Solid Edge part; units mm, degrees
sketch "Sketch1" plane through (0, 0, 0) normal (0, 0, 1) x (1, 0, 0)
  line L0 (0, 0) -> (-71.445, 0)
  line L1 (-40, -28.2156) -> (-71.445, 0)
  line L2 (-40, -52.2156) -> (-40, -28.2156)
  line L3 (-40, -52.2156) -> (-25, -52.2156)
  line L4 (-25, -52.2156) -> (-25, -165)
  line L5 (-25, -165) -> (0, -165)
  line L6 (0, -165) -> (0, 0)
  dimension "D1" = 40
  dimension "D2" = 25
  dimension "D3" = 40
extrude "Protrusion1" add sketch "Sketch1" along normal blind 12
sketch "Sketch2" plane through (0, -70, 6) normal (1, 0, 0) x (0, 1, 0)
  line L0 (70, 2) -> (-55, -6)
  line L1 (-55, -6) -> (-95, 2)
  dimension "D1" = 70
extrude "Extrusionsausschnitt_1" cut sketch "Sketch2" against normal blind 220 material side at (0, -62.4968, 3.9501)
mirror "Mirror1" about plane through (0, 0, 0) normal (-1, 0, 0) of "Protrusion1", "Extrusionsausschnitt_1"
chamfer "Fase_2" distance 2.5 angle 45 12 edges at (25, -88.6078, 2.3291) (25, -145, 4) (0, -165, 8) (-25, -145, 4) (-25, -88.6078, 2.3291) (-32.5, -52.2156, 4.6582) (32.5, -52.2156, 4.6582) (0, 0, 8) (40, -40.2156, 5.4262) (55.7225, -14.1078, 7.0971) (-40, -40.2156, 5.4262) (-55.7225, -14.1078, 7.0971)
sketch "Sketch3" plane through (0, -82.5, 12) normal (0, 0, 1) x (0, -1, 0)
  circle A0 centre (-76.02, 50) radius 2.5
  circle A1 centre (-61.02, 25) radius 2.5
  circle A2 centre (-61.02, -25) radius 2.5
  circle A3 centre (-76.02, -50) radius 2.5
extrude "Extrusionsausprägung_3" add sketch "Sketch3" along normal blind 9
hole "Bohrung_1" at (37.5, -21.48, 12) direction (0, 0, -1) diameter 3.6 end up to next
hole "Hole1" at (-37.5, -21.48, 12) direction (0, 0, -1) diameter 3.6 end up to next
hole "Hole2" at (-17.5, -11.48, 12) direction (0, 0, -1) diameter 3.6 end up to next
hole "Hole3" at (17.5, -11.48, 12) direction (0, 0, -1) diameter 3.6 end up to next
hole "Bohrung_5" at (-6.25, -32.35, 12) direction (0, 0, -1) diameter 5.8 depth 7
hole "Hole4" at (6.25, -32.35, 12) direction (0, 0, -1) diameter 5.8 depth 7
sketch "Sketch4" plane through (0, -82.5, 8) normal (0, 0, 1) x (0, -1, 0)
  circle A0 centre (-61.02, 37.5) radius 2.75
  circle A1 centre (-71.02, 17.5) radius 2.75
  circle A2 centre (-71.02, -17.5) radius 2.75
  circle A3 centre (-61.02, -37.5) radius 2.75
extrude "Extrusionsausschnitt_3" cut sketch "Sketch4" against normal blind 10
hole "Bohrung_7" at (9, -153.11, 12) direction (0, 0, -1) diameter 3.6 end up to next
hole "Hole5" at (-9, -153.11, 12) direction (0, 0, -1) diameter 3.6 end up to next
hole "Hole6" at (-9, -128.11, 12) direction (0, 0, -1) diameter 3.6 end up to next
hole "Hole7" at (9, -128.11, 12) direction (0, 0, -1) diameter 3.6 end up to next
sketch "Sketch5" plane through (0, -82.5, 6) normal (0, 0, 1) x (0, -1, 0)
  circle A0 centre (45.61, 9) radius 2.75
  circle A1 centre (70.61, 9) radius 2.75
  circle A2 centre (70.61, -9) radius 2.75
  circle A3 centre (45.61, -9) radius 2.75
extrude "Extrusionsausschnitt_4" cut sketch "Sketch5" against normal blind 17.8534
properties part number "49" material "Polyacticacid"
Work out the finished part from the listing and answer in its coordinate system (mm). A direction names the side the tool comes from. Coordinates: 2 decimals unless noted, no trailing zeros. Order: outer loops, then holes, each group sorted by start corner. A loop starts at its lowest first (then second) coordinate and runs counter-clockwise, first axis right, second up. Notation, with made-up numbers: (79, 1.25) - (112, 1.25) arc R24 cw to (112, 19.25) - close; hole circle Ø11 at (-31, 16). An arc over 180 degrees is marked (long way). Put each result on its own line as item: value. Start each with the question number.
1) For faces 1 (the cylindrical face through (-36.67, -24.1, 7.24)), 2 (the cylindrical face through (52.44, -5.94, 16.44)), 3 (the flat face through (-25, -108, 8)), 4 (the flat face through (23.77, -86.91, 3.71)), determine the directions among +Z, -Z, +X, -X, +Y, -Y from which every point of the face is accessible in a straight line to the end or side of a thin tool.
2) Find section C-C (x = 50). Give the vertices of the cut face in (y, z).
3) Find section B-B (y = -21.48). State how many separate pieces and enclosed holes the cut face has, plus the area to 3 significant figures.
4) Find section A-A (x = 17.5). Give the vertices of the cut face in (y, z).
5) Flat-ended cylindrical pins translate along their axes: pin 1 (3 mm diameter, centred on x = 9, y = -153.11, fed in from -Z); pin 2 (12 mm diameter, centred on y = -94, z = 12, fed in from +X); pin 3 (6.5 mm diameter, centred on x = -9, y = -153.11, fed in from -Z); pin 4 (1.5 mm diameter, centred on y = -110.5, z = 6.5, fed in from -X). Find the tip coordinate at first contact, or state that the pin passes through.
6) Find section D-D (y = -77). Give the vertices of the cut face in (x, z).
7) Find the intervals of material crossed by line 1 (X direction, y = -21.48, z = 9.75); line 2 (X direction, y = -21.48, z = 7.6); line 3 (Z direction, x = -13, y = -153.5), in increasing order. Write a range as from..to.
Results list:
1. face 1: -Z
1. face 2: +Z
1. face 3: +Z, -Z, -X, -Y
1. face 4: -Z, +X
2. outline: (-19.24, 9.27) - (-15.89, 6.98) - (-2.49, 7.84) - (0, 10.5) - (0, 12) - (-3.98, 12) - (-3.98, 21) - (-8.98, 21) - (-8.98, 12) - (-19.24, 12) - close
3. separate pieces: 3
3. enclosed holes: 0
3. area: 547 mm^2
4. outline: (-165, 10.5) - (-162.55, 7.51) - (-125, 0) - (-14.23, 7.09) - (-14.23, 8) - (-13.28, 8) - (-13.28, 12) - (-165, 12) - close; (-9.68, 8) - (-8.73, 8) - (-8.73, 7.44) - (-2.49, 7.84) - (0, 10.5) - (0, 12) - (-9.68, 12) - close
5. pin 1: passes through
5. pin 2: stops at x = 25
5. pin 3: stops at z = 4.97
5. pin 4: stops at x = -25
6. outline: (-25, 5.58) - (-22.5, 3.07) - (22.5, 3.07) - (25, 5.58) - (25, 12) - (-25, 12) - close
7. line 1: x = -47.51..-39.3, -35.7..35.7, 39.3..47.51
7. line 2: x = -45.22..-40.25, -34.75..34.75, 40.25..45.22
7. line 3: z = 5.7..12
